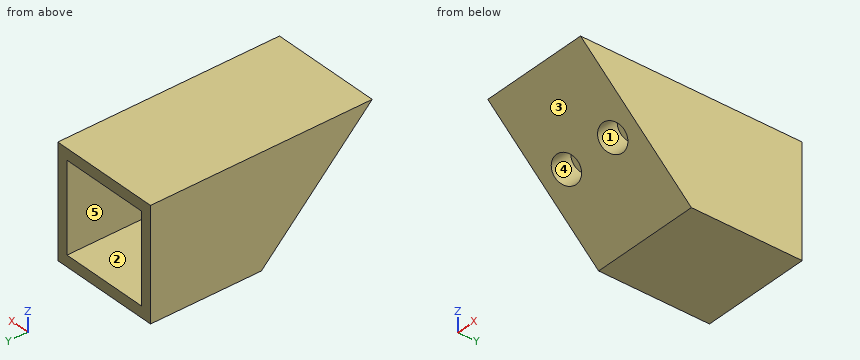
Autodesk Inventor part; units mm, degrees
sketch "Sketch1" plane through (0, 0, 0) normal (1, 0, 0) x (0, 1, 0)
  line L0 (20, 10) -> (-20, 10)
  line L1 (-20, 10) -> (-20, -10)
  line L2 (-20, -10) -> (20, -10)
  line L3 (20, -10) -> (20, 10)
  line L4 (-28, 0) -> (28, 0)
  line L5 (0, 14) -> (0, -14)
  line L6 (0, -10) -> (-20, 10)
  point P0 (0, 0)
  point P1 (20, 0)
  point P2 (0, 10)
  dimension "d0" = 20
  dimension "d1" = 40
extrude "Extrusion1" add sketch "Sketch1" along normal mid plane 20 contours L3 L4 L5 L0 | L5 L4 L6 L0 | L3 L2 L5 L4 | L5 L6 L4
sketch "Sketch2" plane through (-10, 20, 10) normal (0, 1, 0) x (1, 0, 0)
  line L0 (20, 20) -> (0, 20)
  line L1 (20, 20) -> (20, 0)
  line L2 (0, 0) -> (0, 20)
  line L3 (0, 0) -> (20, 0)
  line L4 (2, 18) -> (18, 18)
  line L5 (18, 18) -> (18, 2)
  line L6 (18, 2) -> (2, 2)
  line L7 (2, 2) -> (2, 18)
  point P0 (10, 10)
  dimension "d4" = 2
extrude "Extrusion2" cut sketch "Sketch2" against normal blind 20 contours L4 L5 L6 L7
sketch "Sketch3" plane through (10, 0, -10) normal (0, -0.7071, -0.7071) x (-1, 0, 0)
  line L0 (10, -36.7696) -> (10, 22.6274)
  line L1 (20, -28.2843) -> (0, -28.2843)
  line L2 (10, -28.2843) -> (10, 0)
  line L3 (20, 0) -> (0, 0)
  line L4 (10, -14.1421) -> (20, -14.1421)
  line L5 (20, -28.2843) -> (20, 0)
  line L6 (10, -14.1421) -> (0, -14.1421)
  circle A0 centre (5, -14.1421) radius 2.5
  line L7 (0, -28.2843) -> (0, 0)
  circle A1 centre (15, -14.1421) radius 2.5
  point P0 (10, -7.0711)
  point P1 (0, -14.1421)
  dimension "d8" = 5
  dimension "d9" = 5
extrude "Extrusion3" cut sketch "Sketch3" against normal blind 5 contours A1 L4 | L4 A1 | A0 L6 | L6 A0
properties part number "Chimney"
Geometry: final body of the model. Coordinates: model frame, mm. Face numbers are marked on the shaded views. A direction names the side the tool comes from. Coordinates: 2 decimals unless noted, no trailing zeros. Loops run counter-clockwise (first coordinate to the right, second up) from the corner with the lowest first, then second, coordinate; pieces in that order, holes last. Notation, with made-up numbers: (-39.75, -16) - (-35.75, -16) arc R27 cw to (-35.75, 21) - close; hole circle Ø7 at (74.5, 37.25). An arc over 180 degrees is marked (long way). One line per question, with ' | ' between items. Start each with the question number.
(1) Ray query, L1, parallel to X at y = 16.5, z = -6; L2, parallel to Z at x = 5.25, y = -6. Return the intervals inside material, ascending. Write a range as from..to.
(2) Cut plane C-C on z = -6.25. Output: boundary loops of the cut face in (x, y).
(3) Cut plane A-A on x = 1.75. Output: boundary loops of the cut face in (y, z).
(4) Cut plane B-B on y = 2. Output: boundary loops of the cut face in (x, z), and give its area (3 significant figures).
(5) Cut plane D-D on y = -2.5. Output: boundary loops of the cut face in (x, z).
(6) Draft query along Y for the marked faces 1, 2 and 3. Return one class per face: +Y half, -Y half, draft (parallel to the pull), parting line (faces both ways), or undercut.
(7) Reachability of the marked faces 4 and 5 from +Z, -Z, +X, -X, +Y, -Y: full face, straight path, thin tool, end or side. Return the list, or none.
(8) First-contact query: pin 1 (1.5 mm diameter, centred on x = -5, z = 5, fed in from -Y); pin 2 (1.5 mm diameter, centred on x = -2.5, y = -14.5, fed in from -Z); pin 3 (6 mm diameter, centred on x = 1, y = -10.5, fed in from -Z). Flat tips, straight axial feed; report the tip coordinate or a pass-through.
Here are the results:
1) L1: -10..-8, 8..10 | L2: -4..0.48, 3.07..10
2) outline: (-10, -3.75) - (10, -3.75) - (10, 20) - (8, 20) - (8, 0) - (-8, 0) - (-8, 20) - (-10, 20) - close
3) outline: (-20, 10) - (0, -10) - (20, -10) - (20, -8) - (0, -8) - (0, 8) - (20, 8) - (20, 10) - close
4) outline: (-10, -10) - (10, -10) - (10, 10) - (-10, 10) - close; hole (-8, -8) - (8, -8) - (8, 8) - (-8, 8) - close | area: 144 mm²
5) outline: (-10, -7.5) - (10, -7.5) - (10, 10) - (-10, 10) - close
6) face 1: undercut | face 2: draft | face 3: -Y half
7) face 4: none | face 5: +Y
8) pin 1: y = -15.75 | pin 2: z = 3.75 | pin 3: z = -2.5
